Geometry: final body of the model. Coordinates: model frame, mm. Face numbers are marked on the shaded views. A direction names the side the tool comes from. Coordinates: 2 decimals unless noted, no trailing zeros. Order: outer loops, then holes, each group sorted by start corner. A loop starts at its lowest first (then second) coordinate and runs counter-clockwise, first axis right, second up. Notation, with made-up numbers: M -14.75,76.5 L 41.25,76.5 A27 cw 41.25,115.5 Z; hole C 12,77.25 d11. An arc over 180 degrees is marked long. Use CSV: the item, a comma, the result in double quotes. Start each with the question number.
Q1. Ray query, probe 1 along X at (y, z) = (1.1, 34); probe 2 along Y at (x, z) = (-5.8, 52.5); probe 3 along X at (y, z) = (3.6, -45). Return the intervals inside material, ascending.
Q2. Section query D-D, the plane y = 30. Output: boundary loops of the cut face in (x, z).
Q3. Section query B-B, the plane z = -31. Output: boundary loops of the cut face in (x, y).
Q4. Access query for the marked faces 1, 2 and 3. Directions: +Z, -Z, +X, -X, +Y, -Y. A direction counts if a zero-diameter tool reaches every point of the face in a straight line with its end or side. Return the directions, or none.
Q5. Section query A-A, the plane y = 14.5. Output: boundary loops of the cut face in (x, z).
Q6. Section query C-C, the plane x = 0. State how many separate pieces and enclosed holes the cut face has, and give its area (3 significant figures).
Q7. First-contact query: P1, Ø5, axis at x = -0.5, z = -46, coming from the -Y side; P2, Ø6.5, axis at y = 20, z = 52.5, coming from the +X side; P3, Ø7.5, axis at x = 0, z = -45, coming from the +Y side. Flat tips, straight axial feed; report the tip coordinate or a pass-through.
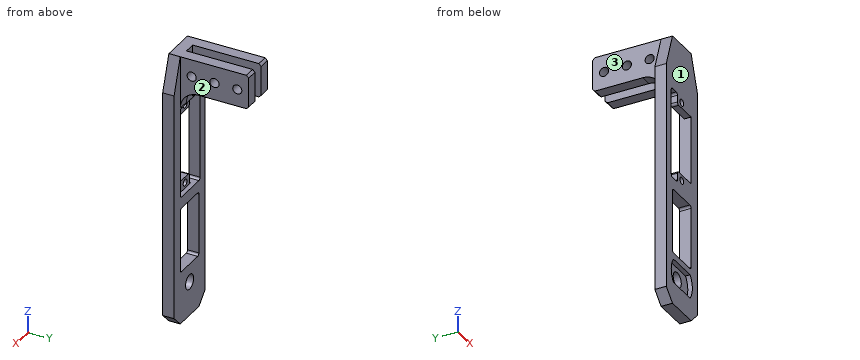
from build123d import *

# Parameters (mm, degrees)
SKETCH1_W           = 25
SKETCH1_H           = 120
BOSS_EXTRUDE1_DEPTH = 5
SKETCH2_W           = 5
SKETCH2_H           = 15
BOSS_EXTRUDE2_DEPTH = 30
CHAMFER1_SIZE       = 5
CHAMFER1_SIZE2      = 15
CHAMFER2_SIZE       = 15
CHAMFER2_SIZE2      = 5
CHAMFER3_SIZE       = 1
CHAMFER4_SIZE       = 5
CUT_EXTRUDE1_DEPTH  = 69.23672032
SKETCH3_3_W         = 11
SKETCH3_3_H         = 5
CUT_EXTRUDE2_DEPTH  = 2
FILLET1_R           = 1
SKETCH4_R           = 1.5
CUT_EXTRUDE3_DEPTH  = 70.139352036
FILLET2_R           = 8
SKETCH6_R           = 3.25
CUT_EXTRUDE5_DEPTH  = 69.23672032
CUT_EXTRUDE6_DEPTH  = 2
SKETCH8_W           = 2
SKETCH8_H           = 2.5
CUT_EXTRUDE7_DEPTH  = 1
SKETCH9_R           = 2
CUT_EXTRUDE8_DEPTH  = 73.284161474
SKETCH10_W          = 15
SKETCH10_H          = 28.5
CUT_EXTRUDE9_DEPTH  = 69.23672032
FILLET3_R           = 1


with BuildPart() as part:
    # Sketch1 → Boss-Extrude1 (new body)
    with BuildSketch(Plane(origin=(0, 0, 0), x_dir=(1, 0, 0), z_dir=(0, 1, 0))):
        Rectangle(SKETCH1_W, SKETCH1_H)
    extrude(amount=BOSS_EXTRUDE1_DEPTH)

    # Sketch2 → Boss-Extrude2 (add)
    with BuildSketch(Plane(origin=(0, 5, 0), x_dir=(1, 0, 0), z_dir=(0, 1, 0))):
        with Locations((-5, -52.5)):
            Rectangle(SKETCH2_W, SKETCH2_H)
        with Locations((5, -52.5)):
            Rectangle(SKETCH2_W, SKETCH2_H)
    extrude(amount=BOSS_EXTRUDE2_DEPTH)

    # Chamfer1
    chamfer1_edges = [part.edges().sort_by_distance(p)[0] for p in [
        (12.5, 2.5, 60),
    ]]
    chamfer1_side = [part.faces().sort_by_distance(p)[0] for p in [
        (-12.069883737, 2.5, 60),
    ]]
    chamfer(chamfer1_edges, length=CHAMFER1_SIZE, length2=CHAMFER1_SIZE2, reference=chamfer1_side[0])

    # Chamfer2
    chamfer2_edges = [part.edges().sort_by_distance(p)[0] for p in [
        (-12.5, 2.5, 60),
    ]]
    chamfer2_side = [part.faces().sort_by_distance(p)[0] for p in [
        (-12.5, 2.5, 0),
    ]]
    chamfer(chamfer2_edges, length=CHAMFER2_SIZE, length2=CHAMFER2_SIZE2, reference=chamfer2_side[0])

    # Chamfer3
    chamfer3_edges = [part.edges().sort_by_distance(p)[0] for p in [
        (-5, 35, 45),
        (-5, 35, 60),
        (5, 35, 45),
        (5, 35, 60),
    ]]
    chamfer(chamfer3_edges, length=CHAMFER3_SIZE)

    # Chamfer4
    chamfer4_edges = [part.edges().sort_by_distance(p)[0] for p in [
        (-12.5, 2.5, -60),
        (12.5, 2.5, -60),
    ]]
    chamfer(chamfer4_edges, length=CHAMFER4_SIZE)

    # Sketch3 → Cut-Extrude1 (cut, through all)
    with BuildSketch(Plane(origin=(0, 5, 0), x_dir=(1, 0, 0), z_dir=(0, 1, 0))):
        Polygon((-8.5, 3.5), (-8.5, -36.5), (-3.5, -36.5), (-3.5, -31.5), (7.5, -31.5), (7.5, -1.5), (-3.5, -1.5), (-3.5, 3.5), align=None)
    extrude(amount=-CUT_EXTRUDE1_DEPTH, mode=Mode.SUBTRACT)

    # Sketch3_3 → Cut-Extrude2 (cut)
    with BuildSketch(Plane(origin=(0, 5, 0), x_dir=(1, 0, 0), z_dir=(0, 1, 0))):
        with Locations((2, 1)):
            Rectangle(SKETCH3_3_W, SKETCH3_3_H)
        with Locations((2, -34)):
            Rectangle(SKETCH3_3_W, SKETCH3_3_H)
    extrude(amount=-CUT_EXTRUDE2_DEPTH, mode=Mode.SUBTRACT)

    # Fillet1
    fillet1_edges = [part.edges().sort_by_distance(p)[0] for p in [
        (-3.5, 1.5, 31.5),
        (-3.5, 1.5, 36.5),
        (-8.5, 2.5, 36.5),
        (-8.5, 2.5, -3.5),
        (-3.5, 1.5, -3.5),
        (-3.5, 1.5, 1.5),
        (7.5, 4, -3.5),
        (7.5, 4, 36.5),
    ]]
    fillet(fillet1_edges, radius=FILLET1_R)

    # Sketch4 → Cut-Extrude3 (cut, through all)
    with BuildSketch(Plane(origin=(0, 3, 0), x_dir=(1, 0, 0), z_dir=(0, 1, 0))):
        with Locations(Location((0, 1, 0), (0, 0, 270))):
            Circle(SKETCH4_R)
        with Locations(Location((0, -34, 0), (0, 0, 270))):
            Circle(SKETCH4_R)
    extrude(amount=-CUT_EXTRUDE3_DEPTH, mode=Mode.SUBTRACT)

    # Fillet2
    fillet2_edges = [part.edges().sort_by_distance(p)[0] for p in [
        (-5, 5, 45),
        (5, 5, 45),
    ]]
    fillet(fillet2_edges, radius=FILLET2_R)

    # Sketch6 → Cut-Extrude5 (cut, through all)
    with BuildSketch(Plane(origin=(0, 5, 0), x_dir=(1, 0, 0), z_dir=(0, 1, 0))):
        with Locations(Location((0, 45, 0), (0, 0, 270))):
            Circle(SKETCH6_R)
    extrude(amount=-CUT_EXTRUDE5_DEPTH, mode=Mode.SUBTRACT)

    # Sketch7 → Cut-Extrude6 (cut)
    with BuildSketch(Plane.XZ):
        with BuildLine():
            Line((-6.684870979, -39.75), (6.684870979, -39.75))
            ThreePointArc((6.684870979, -39.75), (8.5, -45), (6.684870979, -50.25))
            Line((6.684870979, -50.25), (-6.684870979, -50.25))
            ThreePointArc((-6.684870979, -50.25), (-8.5, -45), (-6.684870979, -39.75))
        make_face()
    extrude(amount=-CUT_EXTRUDE6_DEPTH, mode=Mode.SUBTRACT)

    # Sketch8 → Cut-Extrude7 (cut)
    with BuildSketch(Plane.XZ.offset(-2)):
        with Locations((-7.5, -45)):
            Rectangle(SKETCH8_W, SKETCH8_H)
    extrude(amount=-CUT_EXTRUDE7_DEPTH, mode=Mode.SUBTRACT)

    # Sketch9 → Cut-Extrude8 (cut, through all)
    with BuildSketch(Plane(origin=(7.5, 0, 0), x_dir=(0, 0, -1), z_dir=(1, 0, 0))):
        with Locations((-52.5, 30)):
            Circle(SKETCH9_R)
        with Locations((-52.5, 20)):
            Circle(SKETCH9_R)
        with Locations((-52.5, 10)):
            Circle(SKETCH9_R)
    extrude(amount=-CUT_EXTRUDE8_DEPTH, mode=Mode.SUBTRACT)

    # Sketch10 → Cut-Extrude9 (cut, through all)
    with BuildSketch(Plane(origin=(0, 5, 0), x_dir=(1, 0, 0), z_dir=(0, 1, 0))):
        with Locations((0, 22.75)):
            Rectangle(SKETCH10_W, SKETCH10_H)
    extrude(amount=-CUT_EXTRUDE9_DEPTH, mode=Mode.SUBTRACT)

    # Fillet3
    fillet3_edges = [part.edges().sort_by_distance(p)[0] for p in [
        (-7.5, 2.5, -8.5),
        (-7.5, 2.5, -37),
        (7.5, 2.5, -37),
        (7.5, 2.5, -8.5),
    ]]
    fillet(fillet3_edges, radius=FILLET3_R)


solid = part.part
Responses:
1,probe 1,"x = -12.5 to -8.5, -3.5 to -1.5, 1.5 to 12.5"
1,probe 2,"y = 0 to 8, 12 to 18, 22 to 28, 32 to 35"
1,probe 3,"x = -12.5 to -3.25, 3.25 to 12.5"
2,outline,"M -7.5,45 L -2.5,45 L -2.5,50.5 L -7.5,50.5 Z; M -7.5,54.5 L -2.5,54.5 L -2.5,60 L -7.5,60 Z; M 2.5,45 L 7.5,45 L 7.5,50.5 L 2.5,50.5 Z; M 2.5,54.5 L 7.5,54.5 L 7.5,60 L 2.5,60 Z"
3,outline,"M -12.5,0 L -7.5,0 L -7.5,5 L -12.5,5 Z; M 7.5,0 L 12.5,0 L 12.5,5 L 7.5,5 Z"
4,face 1,"+Z, -Z, +X, -X, -Y"
4,face 2,"+Z, -Z, +X, +Y"
4,face 3,"+Z, -Z, -X, +Y"
5,outline,"M -7.5,45 L -2.5,45 L -2.5,60 L -7.5,60 Z; M 2.5,45 L 7.5,45 L 7.5,60 L 2.5,60 Z"
6,separate pieces,"6"
6,enclosed holes,"0"
6,area,"229 mm²"
7,P1,"stops at y = 2"
7,P2,"stops at x = 7.5"
7,P3,"stops at y = 5"
